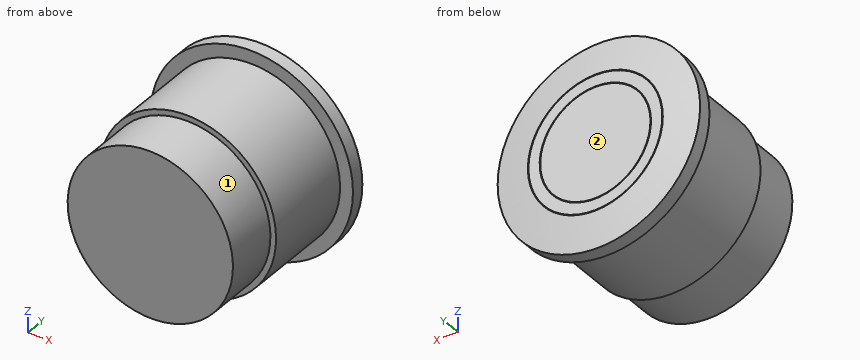
from build123d import *

# Parameters (mm, degrees)
SKETCH1_R           = 7.35
BOSS_EXTRUDE1_DEPTH = 4.8
SKETCH2_R           = 7.85
BOSS_EXTRUDE2_DEPTH = 8.2
SKETCH4_R           = 6
SKETCH4_R_2         = 5.95
SKETCH4_R_3         = 4.95
SKETCH4_R_4         = 4.9
CUT_EXTRUDE1_DEPTH  = 2


with BuildPart() as part:
    # Sketch1 → Boss-Extrude1 (new body)
    with BuildSketch(Plane(origin=(0, 0, 0), x_dir=(1, 0, 0), z_dir=(0, 1, 0))):
        with Locations(Location((0, 0, 0), (0, 0, 270))):
            Circle(SKETCH1_R)
    extrude(amount=BOSS_EXTRUDE1_DEPTH)

    # Sketch2 → Boss-Extrude2 (add)
    with BuildSketch(Plane(origin=(0, 4.8, 0), x_dir=(1, 0, 0), z_dir=(0, 1, 0))):
        with Locations(Location((0, 0, 0), (0, 0, 90))):
            Circle(SKETCH2_R)
    extrude(amount=BOSS_EXTRUDE2_DEPTH)

    # Sketch3 → Revolve2 (revolve)
    with BuildSketch(Plane.XY):
        with BuildLine():
            Line((-9, 13), (-7.85, 13))
            Line((-7.85, 13), (0, 13))
            Line((0, 13), (0, 14.655364075))
            Line((0, 14.655364075), (-6, 14.655364075))
            ThreePointArc((-6, 14.655364075), (-7.503455145, 14.450444998), (-9, 14.2))
            Line((-9, 14.2), (-9, 13))
        make_face()
    revolve(axis=Axis((0, 15.200891001, 0), (0, -1, 0)))

    # Sketch4 → Cut-Extrude1 (cut)
    # profile 1 of 2: a face of its own
    with BuildSketch(Plane(origin=(0, 14.655364075, 0), x_dir=(1, 0, 0), z_dir=(0, 1, 0))):
        with Locations(Location((0, 0, 0), (0, 0, 270))):
            Circle(SKETCH4_R)
        with Locations(Location((0, 0, 0), (0, 0, 270))):
            Circle(SKETCH4_R_2, mode=Mode.SUBTRACT)
    # profile 2 of 2: a face of its own
    with BuildSketch(Plane(origin=(0, 14.655364075, 0), x_dir=(1, 0, 0), z_dir=(0, 1, 0))):
        with Locations(Location((0, 0, 0), (0, 0, 270))):
            Circle(SKETCH4_R_3)
        with Locations(Location((0, 0, 0), (0, 0, 270))):
            Circle(SKETCH4_R_4, mode=Mode.SUBTRACT)
    extrude(amount=-CUT_EXTRUDE1_DEPTH, mode=Mode.SUBTRACT)


solid = part.part
Input: part model. Units: mm. Frame: model coordinates. Face numbers are marked on the shaded views. A direction names the side the tool comes from. Give positions to 0.01 mm unless a question says otherwise; leave off trailing zeros. Order: outer loops, then holes, each group sorted by start corner. A loop starts at its lowest first (then second) coordinate and runs counter-clockwise, first axis right, second up. Notation, with made-up numbers: (62.5, -2.5) - (110.5, -2.5) arc R22 cw to (110.5, 22.5) - close; hole circle Ø8 at (58, 43). An arc over 180 degrees is marked (long way). Answer as a JSON object with one key per item and string values. Group by question number.
Q1. Cut plane C-C, the plane x = 0. Output: boundary loops of the cut face in (y, z), then the cut area to 3 significant figures.
Q2. First-contact query: pin 1 Ø1 at (x, z) = (6.5, -2.5) entering from +Y; pin 2 Ø5 at (x, y) = (4, 8) entering from +Z; pin 3 Ø4 at (y, z) = (2.5, -6) entering from +X. Flat tips, straight axial feed; report the tip coordinate or a pass-through.
Q3. Line query: probe 1 along X at (y, z) = (2.5, -4.25); probe 2 along X at (y, z) = (5.75, 7); probe 3 along Y at (x, z) = (4.5, 7.5). Output: solid intervals per line, ascending.
Q4. Set-up query: the marked faces 1 and 2. Return all of +Z, -Z, +X, -X, +Y, -Y with unobstructed straight access to the full face (end or side cutting, diameter ignored); none if empty.
Q5. Cut plane A-A, the plane y = 13.5. Output: boundary loops of the cut face in (x, z), then the cut area to 3 significant figures.
Q6. Cut plane D-D, the plane y = 5.75. Output: boundary loops of the cut face in (x, z).
Q7. Cut plane B-B, the plane z = 0. Output: boundary loops of the cut face in (x, y), then the cut area to 3 significant figures.
Results:
{
 "1": {"outline": "(0, -7.35) - (4.8, -7.35) - (4.8, -7.85) - (13, -7.85) - (13, -9) - (14.2, -9) arc R50 ccw to (14.66, -6) - (12.66, -6) - (12.66, -5.95) - (14.66, -5.95) - (14.66, -4.95) - (12.66, -4.95) - (12.66, -4.9) - (14.66, -4.9) - (14.66, 4.9) - (12.66, 4.9) - (12.66, 4.95) - (14.66, 4.95) - (14.66, 5.95) - (12.66, 5.95) - (12.66, 6) - (14.66, 6) arc R50 ccw to (14.2, 9) - (13, 9) - (13, 7.85) - (4.8, 7.85) - (4.8, 7.35) - (0, 7.35) - close", "area": "227 mm^2"},
 "2": {"pin 1": "y = 14.6", "pin 2": "z = 7.71", "pin 3": "x = 6.17"},
 "3": {"probe 1": "-6 to 6", "probe 2": "-3.55 to 3.55", "probe 3": "13 to 14.25"},
 "4": {"face 1": "-Y", "face 2": "+Z, -Z, +X, -X, +Y"},
 "5": {"outline": "circle Ø18 at (0, 0); circle Ø11.9 at (0, 0); circle Ø9.8 at (0, 0); hole circle Ø12 at (0, 0); hole circle Ø9.9 at (0, 0)", "area": "251 mm^2"},
 "6": {"outline": "circle Ø15.7 at (0, 0)"},
 "7": {"outline": "(-9, 13) - (-7.85, 13) - (-7.85, 4.8) - (-7.35, 4.8) - (-7.35, 0) - (7.35, 0) - (7.35, 4.8) - (7.85, 4.8) - (7.85, 13) - (9, 13) - (9, 14.2) arc R50 ccw to (6, 14.66) - (6, 12.66) - (5.95, 12.66) - (5.95, 14.66) - (4.95, 14.66) - (4.95, 12.66) - (4.9, 12.66) - (4.9, 14.66) - (-4.9, 14.66) - (-4.9, 12.66) - (-4.95, 12.66) - (-4.95, 14.66) - (-5.95, 14.66) - (-5.95, 12.66) - (-6, 12.66) - (-6, 14.66) arc R50 ccw to (-9, 14.2) - close", "area": "227 mm^2"}
}
